Design review of the part built by this model. Coordinates are the model's own, in mm. A direction names the side the tool comes from. Round coordinates to 2 decimals unless told otherwise and drop trailing zeros. Order: outer loops, then holes, each group sorted by start corner. A loop starts at its lowest first (then second) coordinate and runs counter-clockwise, first axis right, second up. Notation, with made-up numbers: M -26.5,-31.75 L 15.5,-31.75 A15 ccw 15.5,-12.75 Z; hole C -19,18 d4. An arc over 180 degrees is marked long. Use a Markdown table: item, result. Add a question column.
(1) To check wall thickness, follow probe 1 along X at (y, z) = (-140, 7); probe 2 along Y at (x, z) = (-110, 1); probe 3 along X at (y, z) = (-126, 5.5). State the ranges of each line that lie inside material, in increasing order. Write a range as from..to.
(2) Take a section at A-A (x = -110). Write out the cut boundary in (y, z).
(3) Take a section at B-B (y = -140). Write out the cut boundary in (x, z).
(4) The part is to be moulded in two halves that separate along Y. For faces 1 (the face through (-69, -86, 12)), 2 (the face through (-103, -20, 4)), 3 (the face through (-30.33, -142.48, 5.92)), say which applies: released by +Y, released by -Y, zero draft, split by the parting line, or undercut.
(5) Take a section at C-C (x = -87.5). Write out the cut boundary in (y, z).
(6) Take a section at D-D (z = 7.5). Count the separate pieces of the cut face and the enclosed holes in it, then the cut area to 3 significant figures.
(7) Machinability: for faces 4 (the face through (-110, -86, -4)), 5 (the face through (-65, -130, 6)), 6 (the face through (-54, -104, 0)), which of the approach directions +Z, -Z, +X, -X, +Y, -Y give a long, thin tool a straight path to every point of the face, cutting with its end or side? Answer none if there is none.
(8) For pin 1 (24 mm diameter, centred on x = -54, y = -61, fed in from -Z); pin 2 (3.5 mm diameter, centred on x = -72, z = 3, fed in from +Y); pin 3 (6.5 mm diameter, centred on x = -30, y = -140, fed in from -Z); pin 4 (6 mm diameter, centred on x = -110, y = -30, fed in from -Z), all flat-tipped, find the tip position at first contact; note any pin that passes through.
```python
from build123d import *

# Parameters (mm, degrees)
F1_DEPTH  = 12
F2_W      = 100
F2_H      = 20
F3_DEPTH  = 5
F4_W      = 135
F4_H      = 20
F5_DEPTH  = 5
F7_R      = 2.5
F8_DEPTH  = 25
F9_DEPTH  = 5
F10_W     = 20
F10_H     = 20
F10_W_2   = 100
F10_H_2   = 130
F11_DEPTH = 25
F12_W     = 130
F12_H     = 9
F13_DEPTH = 100.0010001
F15_DEPTH = 12.0010001
F16_W     = 80
F16_H     = 4
F17_DEPTH = 20


with BuildPart() as f1:
    # F0 (on Top) → F1 (new body)
    with BuildSketch(Plane.XY):
        with BuildLine():
            add(Edge.make_bspline(
                [(-86.5, 0), (-86.5, -116.5), (0, -116.5)],
                knots=[1.5707963268, 1.5707963268, 1.5707963268, 3.1415926536, 3.1415926536, 3.1415926536], degree=2, weights=[1, 0.7071067812, 1]))
            Line((-86.5, 0), (-86.5, -116.5))
            Line((-86.5, -116.5), (0, -116.5))
        make_face()
        Polygon((-86.5, -116.5), (-86.5, 0), (-100, 0), (-100, -130), (0, -130), (0, -116.5), align=None)
    extrude(amount=F1_DEPTH)

    # F2 (on face) → F3 (join)
    with BuildSketch(Plane.XZ.offset(130)):
        with Locations((-50, 6)):
            Rectangle(F2_W, F2_H)
    extrude(amount=F3_DEPTH)

    # F4 (on face) → F5 (join)
    with BuildSketch(Plane(origin=(-100, 0, 0), x_dir=(0, -1, 0), z_dir=(-1, 0, 0))):
        with Locations((67.5, 6)):
            Rectangle(F4_W, F4_H)
    extrude(amount=F5_DEPTH)

    # F7 (on face) → F8 (join)
    with BuildSketch(Plane(origin=(0, 0, -4), x_dir=(1, 0, 0), z_dir=(0, 0, -1))):
        Polygon((0, 135), (0, 150), (-120, 150), (-120, 0), (-105, 0), (-105, 135), align=None)
        with Locations((-110, 30)):
            Circle(F7_R, mode=Mode.SUBTRACT)
        with Locations((-110, 105)):
            Circle(F7_R, mode=Mode.SUBTRACT)
        with Locations((-80, 140)):
            Circle(F7_R, mode=Mode.SUBTRACT)
        with Locations((-30, 140)):
            Circle(F7_R, mode=Mode.SUBTRACT)
    extrude(amount=-F8_DEPTH)

    # F6 (on face) → F9 (join)
    with BuildSketch(Plane.XY.offset(16)):
        Polygon((-90, 0), (-105, 0), (-105, -135), (0, -135), (0, -120), (-90, -120), align=None)
    extrude(amount=F9_DEPTH)

    # F10 (on Top) → F11 (cut, symmetric)
    with BuildSketch(Plane.XY):
        with Locations((-10, -10)):
            Rectangle(F10_W, F10_H)
        with Locations((-70, -10)):
            Rectangle(F10_W_2, F10_H)
        with Locations((-10, -85)):
            Rectangle(F10_W, F10_H_2)
    extrude(amount=F11_DEPTH, both=True, mode=Mode.SUBTRACT)

    # F12 (on face) → F13 (cut, through all)
    with BuildSketch(Plane.YZ.offset(-20)):
        with Locations((-85, 16.5)):
            Rectangle(F12_W, F12_H)
    extrude(amount=-F13_DEPTH, mode=Mode.SUBTRACT)

    # F14 (on face) → F15 (cut, through all)
    with BuildSketch(Plane(origin=(0, 0, 0), x_dir=(1, 0, 0), z_dir=(0, 0, -1))):
        with BuildLine():
            Line((-30, 130), (-100, 130))
            Line((-100, 130), (-100, 30))
            Line((-100, 30), (-95.2158076494, 30))
            ThreePointArc((-95.2158076494, 30), (-75.8232238431, 85.9047045014), (-30, 123.3431933691))
            Line((-30, 123.3431933691), (-30, 130))
        make_face()
    extrude(amount=-F15_DEPTH, mode=Mode.SUBTRACT)

    # F16 (on face) → F17 (cut, through all)
    with BuildSketch(Plane(origin=(0, -130, 0), x_dir=(-1, 0, 0), z_dir=(0, 1, 0))):
        with Locations((60, -2)):
            Rectangle(F16_W, F16_H)
    extrude(amount=-F17_DEPTH, mode=Mode.SUBTRACT)


solid = f1.part
```
Verdict:
| question | item | result |
|---|---|---|
| 1 | probe 1 | x = -120..-82.5, -77.5..-32.5, -27.5..-20 |
| 1 | probe 2 | y = -150..-107.5, -102.5..-32.5, -27.5..-20 |
| 1 | probe 3 | x = -120..-100, -30..-20 |
| 2 | outline | M -150,-4 L -107.5,-4 L -107.5,12 L -150,12 Z; M -102.5,-4 L -32.5,-4 L -32.5,12 L -102.5,12 Z; M -27.5,-4 L -20,-4 L -20,12 L -27.5,12 Z |
| 3 | outline | M -120,-4 L -100,-4 L -100,0 L -82.5,0 L -82.5,12 L -120,12 Z; M -77.5,0 L -32.5,0 L -32.5,12 L -77.5,12 Z; M -27.5,0 L -20,0 L -20,12 L -27.5,12 Z |
| 4 | face 1 | zero draft |
| 4 | face 2 | released by +Y |
| 4 | face 3 | undercut |
| 5 | outline | M -150,0 L -130,0 L -130,12 L -150,12 Z; M -64.37,0 L -20,0 L -20,12 L -64.37,12 Z |
| 6 | separate pieces | 1 |
| 6 | enclosed holes | 5 |
| 6 | area | 5,920 mm^2 |
| 7 | face 4 | -Z, +X, -X, +Y, -Y |
| 7 | face 5 | +Z, -Z |
| 7 | face 6 | -Z, +X, +Y, -Y |
| 8 | pin 1 | passes through |
| 8 | pin 2 | stops at y = -60.88 |
| 8 | pin 3 | stops at z = 0 |
| 8 | pin 4 | stops at z = -4 |
